```python
from build123d import *

# Parameters (mm, degrees)
ESQUISSE1_W             = 80
ESQUISSE1_H             = 80
ESQUISSE1_R             = 2.5
BOSS_EXTRU_1_DEPTH      = 10
ESQUISSE2_R             = 4.6
ENL_V_MAT_EXTRU_1_DEPTH = 7
ENL_V_MAT_EXTRU_2_DEPTH = 7.5
ESQUISSE5_R             = 4.6
BOSS_EXTRU_2_DEPTH      = 3.5
SYM_TRIE4_COPY_1_DEPTH  = 7.5


with BuildPart() as part:
    # Esquisse1 → Boss.-Extru.1 (new body)
    with BuildSketch(Plane.XY):
        Rectangle(ESQUISSE1_W, ESQUISSE1_H)
        with Locations((-32.5, 20)):
            Circle(ESQUISSE1_R, mode=Mode.SUBTRACT)
        with Locations((-32.5, -20)):
            Circle(ESQUISSE1_R, mode=Mode.SUBTRACT)
        with Locations((32.5, -20)):
            Circle(ESQUISSE1_R, mode=Mode.SUBTRACT)
        with Locations((32.5, 20)):
            Circle(ESQUISSE1_R, mode=Mode.SUBTRACT)
    extrude(amount=BOSS_EXTRU_1_DEPTH)

    # Esquisse2 → Enlèv. mat.-Extru.1 (cut)
    with BuildSketch(Plane.XY.offset(10)):
        with Locations((-32.5, 20)):
            Circle(ESQUISSE2_R)
        with Locations(Location((-32.5, -20, 0), (0, 0, 180))):
            Circle(ESQUISSE2_R)
        with Locations((32.5, -20)):
            Circle(ESQUISSE2_R)
        with Locations(Location((32.5, 20, 0), (0, 0, 180))):
            Circle(ESQUISSE2_R)
    extrude(amount=-ENL_V_MAT_EXTRU_1_DEPTH, mode=Mode.SUBTRACT)

    # Esquisse4 → Enlèv. mat.-Extru.2 (cut)
    with BuildSketch(Plane.ZY.offset(40)):
        Polygon((6.5, 24.6), (6.5, 15.4), (3, 15.4), (3, 17.5), (0, 17.5), (0, 22.5), (3, 22.5), (3, 24.6), align=None)
    enl_v_mat_extru_2 = extrude(amount=-ENL_V_MAT_EXTRU_2_DEPTH, mode=Mode.SUBTRACT)

    # Symétrie1: Enlèv. mat.-Extru.2 across plane
    add(enl_v_mat_extru_2.mirror(Plane.ZX), mode=Mode.SUBTRACT)

    # Esquisse5 → Boss.-Extru.2 (add)
    with BuildSketch(Plane.XY.offset(10)):
        with Locations((-32.5, 20)):
            Circle(ESQUISSE5_R)
        with Locations(Location((32.5, 20, 0), (0, 0, 90))):
            Circle(ESQUISSE5_R)
        with Locations((32.5, -20)):
            Circle(ESQUISSE5_R)
        with Locations((-32.5, -20)):
            Circle(ESQUISSE5_R)
    extrude(amount=-BOSS_EXTRU_2_DEPTH)

    # Symétrie4: Enlèv. mat.-Extru.2 across plane
    add(enl_v_mat_extru_2.mirror(Plane(origin=(0, 0, 0), x_dir=(0, 0, 1), z_dir=(1, 0, 0))), mode=Mode.SUBTRACT)

    # Symétrie4 copy 1 sketch → Symétrie4 copy 1 (cut)
    with BuildSketch(Plane(origin=(40, 0, 0), x_dir=(0, 0, 1), z_dir=(1, 0, 0))):
        Polygon((6.5, 24.6), (6.5, 15.4), (3, 15.4), (3, 17.5), (0, 17.5), (0, 22.5), (3, 22.5), (3, 24.6), align=None)
    extrude(amount=-SYM_TRIE4_COPY_1_DEPTH, mode=Mode.SUBTRACT)


solid = part.part
```
Verification items for the finished model (mm, model axes). A direction names the side the tool comes from. Round coordinates to 2 decimals unless told otherwise and drop trailing zeros. Write each loop counter-clockwise with the first axis right and the second up, starting at its lowest first coordinate (ties: lowest second). Pieces come first, ordered by that corner, then holes.
1. Section check D-D on z = 1. Enter the section's corners in (x, y), plus the area to 3 significant figures.
2. Access from +Z, -Z, +X, -X, +Y, -Y to the whole of each face (thin tool, end or side, straight path). Record for faces 1 (the cylindrical face through (30, -20, 1)), 2 (the flat face through (-36, 22.5, 1)), 3 (the flat face through (34, -17, 3)).
3. Section check C-C on x = 29. Enter the section's corners in (y, z), plus the area to 3 significant figures.
4. Section check A-A on z = 5. Enter the section's corners in (x, y), plus the area to 3 significant figures.
5. Draft check along Y on faces 4 (the flat face through (-1, 1, 0)), 5 (the cylindrical face through (-27.9, 19.9, 4.8)), 6 (the flat face through (-1, 40, 5)). Enter one of: +Y half, -Y half, draft (parallel to the pull), parting line (faces both ways), or undercut.
6. Section check B-B on y = -20. Enter the section's corners in (x, z).
7. Scan lines: L1, parallel to Z at x = 34.5, y = 23.5; L2, parallel to Z at x = -31, y = -20; L3, parallel to X at y = -21.5, z = 1. Record each from-to range of solid material in increasing order.
Answer:
1. outline: (-40, -40) - (40, -40) - (40, -22.5) - (32.5, -22.5) arc R2.5 cw to (32.5, -17.5) - (40, -17.5) - (40, 17.5) - (32.5, 17.5) arc R2.5 cw to (32.5, 22.5) - (40, 22.5) - (40, 40) - (-40, 40) - (-40, 22.5) - (-32.5, 22.5) arc R2.5 cw to (-32.5, 17.5) - (-40, 17.5) - (-40, -17.5) - (-32.5, -17.5) arc R2.5 cw to (-32.5, -22.5) - (-40, -22.5) - close
1. area: 6,210 mm2
2. face 1: -Z, +X
2. face 2: -Z, -X
2. face 3: +X
3. outline: (-40, 0) - (40, 0) - (40, 10) - (-40, 10) - close; hole (-22.98, 3) - (-17.02, 3) - (-17.02, 6.5) - (-22.98, 6.5) - close; hole (17.02, 3) - (22.98, 3) - (22.98, 6.5) - (17.02, 6.5) - close
3. area: 758 mm2
4. outline: (-40, -40) - (40, -40) - (40, -24.6) - (32.5, -24.6) arc R4.6 cw to (32.5, -15.4) - (40, -15.4) - (40, 15.4) - (32.5, 15.4) arc R4.6 cw to (32.5, 24.6) - (40, 24.6) - (40, 40) - (-40, 40) - (-40, 24.6) - (-32.5, 24.6) arc R4.6 cw to (-32.5, 15.4) - (-40, 15.4) - (-40, -15.4) - (-32.5, -15.4) arc R4.6 cw to (-32.5, -24.6) - (-40, -24.6) - close
4. area: 5,990 mm2
5. face 4: draft
5. face 5: undercut
5. face 6: +Y half
6. outline: (-40, 6.5) - (-27.9, 6.5) - (-27.9, 3) - (-30, 3) - (-30, 0) - (30, 0) - (30, 3) - (27.9, 3) - (27.9, 6.5) - (40, 6.5) - (40, 10) - (-40, 10) - close
7. L1: z = 0 to 3, 6.5 to 10
7. L2: z = 6.5 to 10
7. L3: x = -30.5 to 30.5
